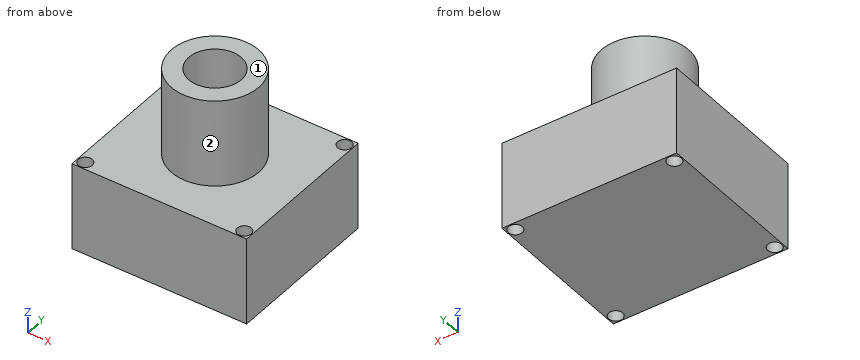
Autodesk Inventor part; units mm, degrees
ref_plane "YZ Plane" through (0, 0, 0) normal (1, 0, 0) x (0, 1, 0)
ref_plane "XZ Plane" through (0, 0, 0) normal (0, 1, 0) x (-1, 0, 0)
ref_plane "XY Plane" through (0, 0, 0) normal (0, 0, 1) x (1, 0, 0)
sketch "Sketch1" plane through (0, 0, 0) normal (0, 0, 1) x (1, 0, 0)
  line L0 (-50, 45) -> (50, 45)
  line L1 (50, 45) -> (50, -45)
  line L2 (50, -45) -> (-50, -45)
  line L3 (-50, -45) -> (-50, 45)
  line L4 (-50, 45) -> (50, -45) construction
  line L5 (50, 45) -> (-50, -45) construction
  point P0 (0, 0)
extrude "Extrusion1" add sketch "Sketch1" against normal blind 50
sketch "Sketch2" plane through (0, 0, 0) normal (0, 0, 1) x (1, 0, 0)
  circle A0 centre (0, 0) radius 25
extrude "Extrusion2" add sketch "Sketch2" along normal blind 50
sketch "Sketch3" plane through (0, 0, 50) normal (0, 0, 1) x (1, 0, 0)
  circle A0 centre (0, 0) radius 15
extrude "Extrusion3" cut sketch "Sketch3" against normal blind 30
thread "Thread1"
sketch "Sketch4" plane through (0, 0, 0) normal (0, 0, 1) x (1, 0, 0)
  line L0 (-50, 45) -> (50, 45)
  line L1 (-50, 45) -> (-41, 45)
  line L2 (-50, 36) -> (-50, 45)
  line L3 (50, 45) -> (41, 45)
  line L4 (50, 36) -> (50, 45)
  line L5 (50, -45.06) -> (41, -45.06)
  line L6 (50, -36.06) -> (50, -45.06)
  line L7 (-50, -45.06) -> (-41, -45.06)
  line L8 (-50, -36.06) -> (-50, -45.06)
  circle A0 centre (-45.5, 40.5) radius 4
  circle A1 centre (45.5, 40.5) radius 4
  circle A2 centre (45.5, -40.56) radius 4
  circle A3 centre (-45.5, -40.56) radius 4
  point P0 (0, 0)
extrude "Extrusion4" cut sketch "Sketch4" against normal through all
equation "\"BendRadius\" = Thickness"
equation "\"BendReliefWidth\" = Thickness"
equation "\"BendReliefDepth\" = 0.5 * Thickness"
equation "\"CornerReliefSize\" = 4 * Thickness"
equation "\"MinimumRemnant\" = 2 * Thickness"
equation "\"TransitionRadius\" = BendRadius"
equation "\"JacobiRadiusSize\" = BendRadius"
equation "\"GapSize\" = Thickness"
properties part number "Practica 1 Sofia Lopez"
Build history of the part. All positions in model axes, mm. Face numbers are marked on the shaded views. A direction names the side the tool comes from. Give positions to 0.01 mm unless a question says otherwise; leave off trailing zeros. Loops run counter-clockwise (first coordinate to the right, second up) from the corner with the lowest first, then second, coordinate; pieces in that order, holes last.
Item 1: Slice it at B-B, the plane x = 45.5. List the corners of the cut face in (y, z).
Answers follow:
outline: (-45, -50) - (-44.56, -50) - (-44.56, 0) - (-45, 0) - close; (-36.56, -50) - (36.5, -50) - (36.5, 0) - (-36.56, 0) - close; (44.5, -50) - (45, -50) - (45, 0) - (44.5, 0) - close
Item 2: Flat gauge pins, fed straight in: pin 1 (9 mm diameter, centred on x = -45.5, y = 40.5, fed in from +Z); pin 2 (5 mm diameter, centred on x = -9, z = 24.5, fed in from -Y); pin 3 (6 mm diameter, centred on x = -16, z = 5, fed in from +Y). Where does each tip first touch, or does it go through?
Answers follow:
pin 1: stops at z = 0
pin 2: stops at y = -24.14
pin 3: stops at y = 21.35
Item 3: Which spindle directions (+Z, -Z, +X, -X, +Y, -Y) get a long thin tool onto all of the face, cutting with end or side? Do the marked faces 1 and 2. Say none if no direction does.
Answers follow:
face 1: +Z, +X, -X, +Y, -Y
face 2: +Z
Item 4: Slice it at D-D, the plane y = 0. List the corners of the cut face in (x, z), and give its area (3 significant figures).
Answers follow:
outline: (-50, -50) - (50, -50) - (50, 0) - (25, 0) - (25, 50) - (15, 50) - (15, 20) - (-15, 20) - (-15, 50) - (-25, 50) - (-25, 0) - (-50, 0) - close
area: 6,600 mm2
Item 5: Slice it at A-A, the plane y = 40.5. List the corners of the cut face in (x, z), and give its area (3 significant figures).
Answers follow:
outline: (-50, -50) - (-49.5, -50) - (-49.5, 0) - (-50, 0) - close; (-41.5, -50) - (41.5, -50) - (41.5, 0) - (-41.5, 0) - close; (49.5, -50) - (50, -50) - (50, 0) - (49.5, 0) - close
area: 4,200 mm2
Item 6: Drill centre lines: line 1 (Y direction, x = -45, z = -13); line 2 (X direction, y = 40, z = -12); line 3 (X direction, y = 39.5, z = -15). Where is each one in solid material? Low to high.
Answers follow:
line 1: y = -45 to -44.53, -36.59 to 36.53, 44.47 to 45
line 2: x = -50 to -49.47, -41.53 to 41.53, 49.47 to 50
line 3: x = -50 to -49.37, -41.63 to 41.63, 49.37 to 50
Item 7: Slice it at C-C, the plane z = -17.5. List the corners of the cut face in (x, y), and give its area (3 significant figures).
Answers follow:
outline: (-50, -45) - (50, -45) - (50, 45) - (-50, 45) - close; hole circle Ø8 at (-45.5, -40.56); hole circle Ø8 at (-45.5, 40.5); hole circle Ø8 at (45.5, -40.56); hole circle Ø8 at (45.5, 40.5)
area: 8,800 mm2
